Build history of the part. All positions in model axes, mm. A direction names the side the tool comes from. Round coordinates to 2 decimals unless told otherwise and drop trailing zeros. Loops run counter-clockwise (first coordinate to the right, second up) from the corner with the lowest first, then second, coordinate; pieces in that order, holes last.
from build123d import *


with BuildPart() as part:
    # Sketch1 → Revolve1 (revolve)
    with BuildSketch(Plane(origin=(0, 0, 0), x_dir=(1, 0, 0), z_dir=(0, 1, 0)), mode=Mode.PRIVATE) as revolve1_sk:
        Polygon((0, 23.5), (0, 15), (32, 15), (32, 22), (34, 22), (34, 23.5), align=None)
    revolve(revolve1_sk.sketch.rotate(Axis((0, 0, 0), (1, 0, 0)), 180), axis=Axis((0, 0, 0), (1, 0, 0)))

    # Sketch7 → Groove for DIN 471 - 45 x 1.75, Circlip for shafts - normal1 (revolve, cut)
    with BuildSketch(Plane(origin=(0, 0, 0), x_dir=(0, 0, 1), z_dir=(0, -1, 0))):
        with BuildLine():
            Line((21.435, -23.95), (28.2, -23.95))
            Line((28.2, -23.95), (28.2, -22.1))
            Line((28.2, -22.1), (21.435, -22.1))
            ThreePointArc((21.435, -22.1), (21.304185245, -22.154185245), (21.25, -22.285))
            Line((21.25, -22.285), (21.25, -23.765))
            ThreePointArc((21.25, -23.765), (21.304185245, -23.895814755), (21.435, -23.95))
        make_face()
    revolve(axis=Axis((50, 0, 0), (-1, 0, 0)), mode=Mode.SUBTRACT)

    # Mirror2: part across plane


with BuildPart() as part_1:
    add(part.part)
    add(part.part.mirror(Plane.ZY))


solid = part_1.part
(1) Pull direction X, two halves, no side cores. Call faces 1 (the face through (32, -5.2, -14.4)), 2 (the face through (23.035, -12.93, -16.863)), 3 (the face through (-32, -5.2, -14.4)): +X half, -X half, draft (parallel to the pull), parting line (faces both ways), or undercut.
Responses:
face 1: +X half
face 2: undercut
face 3: -X half
(2) Pin check, flat tips, straight feed: P1, Ø22, axis at y = -10.5, z = -2.5, coming from the -X side; P2, Ø12, axis at y = -7, z = -10.5, coming from the +X side; P3, Ø4, axis at x = -12.5, y = -9.5, coming from the +Z side. Stop position of each tip, or through.
Responses:
P1: stops at x = -32
P2: stops at x = 32
P3: stops at z = 22.27
(3) Slice it at A-A on x = -18. List the corners of the cut face in (y, z).
Responses:
outline: circle Ø47 at (0, 0); hole circle Ø30 at (0, 0)
(4) Which spindle directions (+Z, -Z, +X, -X, +Y, -Y) get a long thin tool onto all of the face, cutting with end or side? Do faces 4 (the face through (-28.9, -23.3, -3.06)), 5 (the face through (34, 16, -16)), 6 (the face through (-23.95, -21, 5)), 7 (the face through (33.014, 21.477, -4.769)), 8 (the face through (-33.014, 21.477, -4.769)). Say none if no direction does.
Responses:
face 4: +X, -X
face 5: +Z, -Z, +X, +Y, -Y
face 6: none
face 7: +X
face 8: -X
(5) Probe line 1 (Y direction, x = 32.9, z = 0); line 2 (Y direction, x = 11, z = 0); line 3 (X direction, y = 17, z = 9.5). List the from-to ranges inside material, lowest first.
Responses:
line 1: y = -23.5 to -22, 22 to 23.5
line 2: y = -23.5 to -15, 15 to 23.5
line 3: x = -32 to 32
